from build123d import *

# Parameters (mm, degrees)
SKETCH1_W           = 101.6
SKETCH1_H           = 17.78
SKETCH1_R           = 3.96875
BOSS_EXTRUDE1_DEPTH = 33.02
SKETCH2_R           = 2.4892
CUT_EXTRUDE1_DEPTH  = 17.78
SKETCH3_R           = 4.064
CUT_EXTRUDE2_DEPTH  = 4.826
CUT_EXTRUDE3_DEPTH  = 109.300548475
FILLET1_R           = 2.54
SKETCH6_W           = 13.97
SKETCH6_H           = 22.86
SKETCH6_W_2         = 10.94852006
SKETCH6_H_2         = 22.718450652
CUT_EXTRUDE4_DEPTH  = 106.921350067
FILLET2_R           = 2.54
FILLET3_R           = 1.27


with BuildPart() as part:
    # Sketch1 → Boss-Extrude1 (new body)
    with BuildSketch(Plane(origin=(0, 0, 0), x_dir=(1, 0, 0), z_dir=(0, 1, 0))):
        with Locations((50.8, 8.89)):
            Rectangle(SKETCH1_W, SKETCH1_H)
        with Locations(Location((76.2, 8.89, 0), (0, 0, 270))):
            Circle(SKETCH1_R, mode=Mode.SUBTRACT)
        with Locations(Location((25.4, 8.89, 0), (0, 0, 270))):
            Circle(SKETCH1_R, mode=Mode.SUBTRACT)
    extrude(amount=-BOSS_EXTRUDE1_DEPTH)

    # Sketch2 → Cut-Extrude1 (cut)
    with BuildSketch(Plane.XY):
        with Locations((63.5, -16.51)):
            Circle(SKETCH2_R)
        with Locations((12.7, -16.51)):
            Circle(SKETCH2_R)
    extrude(amount=-CUT_EXTRUDE1_DEPTH, mode=Mode.SUBTRACT)

    # Sketch3 → Cut-Extrude2 (cut)
    with BuildSketch(Plane.XY):
        with Locations((63.5, -16.51)):
            Circle(SKETCH3_R)
        with Locations((12.7, -16.51)):
            Circle(SKETCH3_R)
    extrude(amount=-CUT_EXTRUDE2_DEPTH, mode=Mode.SUBTRACT)

    # Sketch5 → Cut-Extrude3 (cut, through all)
    with BuildSketch(Plane.XY):
        with BuildLine():
            Line((12.7, -5.150774674), (12.7, 0))
            Line((12.7, 0), (0, 0))
            Line((0, 0), (0, -33.02))
            Line((0, -33.02), (12.7, -33.02))
            Line((12.7, -33.02), (12.7, -27.869225326))
            ThreePointArc((12.7, -27.869225326), (12.37660211, -27.022558659), (11.571111111, -26.607089178))
            ThreePointArc((11.571111111, -26.607089178), (2.54, -16.51), (11.571111111, -6.412910822))
            ThreePointArc((11.571111111, -6.412910822), (12.37660211, -5.997441341), (12.7, -5.150774674))
        make_face()
        with BuildLine():
            Line((88.9, -5.150774674), (88.9, 0))
            Line((88.9, 0), (101.6, 0))
            Line((101.6, 0), (101.6, -33.02))
            Line((101.6, -33.02), (88.9, -33.02))
            Line((88.9, -33.02), (88.9, -27.869225326))
            ThreePointArc((88.9, -27.869225326), (89.22339789, -27.022558659), (90.028888889, -26.607089178))
            ThreePointArc((90.028888889, -26.607089178), (99.06, -16.51), (90.028888889, -6.412910822))
            ThreePointArc((90.028888889, -6.412910822), (89.22339789, -5.997441341), (88.9, -5.150774674))
        make_face()
    extrude(amount=-CUT_EXTRUDE3_DEPTH, mode=Mode.SUBTRACT)

    # Fillet1
    fillet1_edges = [part.edges().sort_by_distance(p)[0] for p in [
        (12.7, -33.02, -8.89),
        (12.7, 0, -8.89),
        (88.9, 0, -8.89),
        (88.9, -33.02, -8.89),
    ]]
    fillet(fillet1_edges, radius=FILLET1_R)

    # Sketch6 → Cut-Extrude4 (cut, through all)
    with BuildSketch(Plane.XY):
        with BuildLine():
            Line((19.05, -21.9075), (19.05, -11.1125))
            ThreePointArc((19.05, -11.1125), (19.793948776, -9.316448776), (21.59, -8.5725))
            Line((21.59, -8.5725), (31.75, -8.5725))
            Line((31.75, -8.5725), (31.75, -5.08))
            Line((31.75, -5.08), (54.61, -5.08))
            ThreePointArc((54.61, -5.08), (56.406051224, -5.823948776), (57.15, -7.62))
            Line((57.15, -7.62), (57.15, -25.4))
            ThreePointArc((57.15, -25.4), (56.406051224, -27.196051224), (54.61, -27.94))
            Line((54.61, -27.94), (31.75, -27.94))
            Line((31.75, -27.94), (31.75, -24.4475))
            Line((31.75, -24.4475), (21.59, -24.4475))
            ThreePointArc((21.59, -24.4475), (19.793948776, -23.703551224), (19.05, -21.9075))
        make_face()
        with Locations((76.835, -16.51)):
            Rectangle(SKETCH6_W, SKETCH6_H)
        with Locations((94.37426003, -16.51)):
            Rectangle(SKETCH6_W_2, SKETCH6_H_2)
    extrude(amount=-CUT_EXTRUDE4_DEPTH, mode=Mode.SUBTRACT)

    # Fillet2
    fillet2_edges = [part.edges().sort_by_distance(p)[0] for p in [
        (69.85, -5.08, -8.89),
        (83.82, -27.94, -8.89),
        (83.82, -5.08, -8.89),
        (69.85, -27.94, -8.89),
    ]]
    fillet(fillet2_edges, radius=FILLET2_R)

    # Fillet3
    fillet3_edges = [part.edges().sort_by_distance(p)[0] for p in [
        (31.75, -24.4475, -8.89),
        (31.75, -8.5725, -8.89),
        (31.75, -5.08, -8.89),
        (31.75, -27.94, -8.89),
    ]]
    fillet(fillet3_edges, radius=FILLET3_R)


solid = part.part
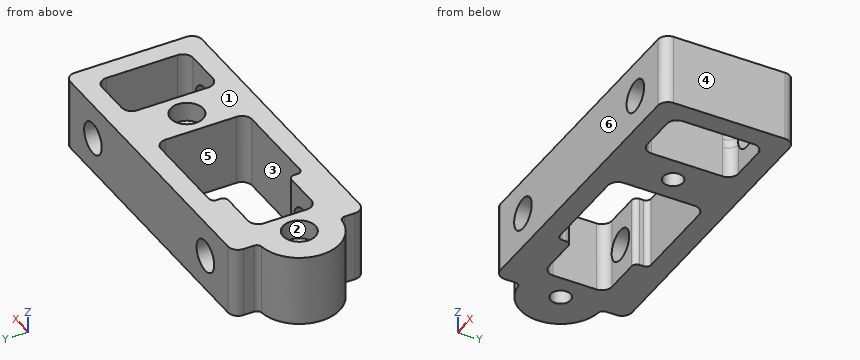
Geometry check sheet. Reference: the model listing, model coordinates, mm. Face numbers are marked on the shaded views. A direction names the side the tool comes from. Give positions to 0.01 mm unless a question says otherwise; leave off trailing zeros. Order: outer loops, then holes, each group sorted by start corner. A loop starts at its lowest first (then second) coordinate and runs counter-clockwise, first axis right, second up. Notation, with made-up numbers: M 88.5,63.5 L 100.5,63.5 A17 ccw 100.5,88.5 Z; hole C -10.5,8.5 d11. An arc over 180 degrees is marked long. Use a Markdown table: item, result.
Item 1: Section check C-C (x = 37.5). Record the cut outline in (y, z), and give its area (3 significant figures).
Answers follow:
| item | result |
|---|---|
| outline | M -33.02,-17.78 L -27.94,-17.78 L -27.94,0 L -33.02,0 Z; M -5.08,-17.78 L 0,-17.78 L 0,0 L -5.08,0 Z |
| area | 181 mm2 |
Item 2: Section check D-D (y = -23.5). Record the cut outline in (x, z), and give its area (3 significant figures).
Answers follow:
| item | result |
|---|---|
| outline | M 5.33,-17.78 L 19.61,-17.78 L 19.61,0 L 5.33,0 Z; M 57.15,-17.78 L 69.85,-17.78 L 69.85,0 L 57.15,0 Z; M 83.82,-17.78 L 88.9,-17.78 L 88.9,0 L 83.82,0 Z |
| area | 570 mm2 |
Item 3: Draft check along X on the marked faces 4, 5 and 6. Enter one of: +X half, -X half, draft (parallel to the pull), parting line (faces both ways), or undercut.
Answers follow:
| item | result |
|---|---|
| face 4 | +X half |
| face 5 | undercut |
| face 6 | draft |
Item 4: Section check A-A (x = 25.4). Record the cut outline in (y, z).
Answers follow:
| item | result |
|---|---|
| outline | M -33.02,-17.78 L -24.45,-17.78 L -24.45,-12.86 L -33.02,-12.86 Z; M -33.02,-4.92 L -24.45,-4.92 L -24.45,0 L -33.02,0 Z; M -8.57,-17.78 L 0,-17.78 L 0,-12.86 L -8.57,-12.86 Z; M -8.57,-4.92 L 0,-4.92 L 0,0 L -8.57,0 Z |
Item 5: Material ranges on line 1 along X through (y, z) = (-28, -8.89); line 2 along X through (y, z) = (-16.5, -6); line 3 along Y through (x, z) = (23.5, -4.5), recorded low to high.
Answers follow:
| item | result |
|---|---|
| line 1 | x = 12.7 to 21.43, 29.37 to 72.23, 80.17 to 88.9 |
| line 2 | x = 2.54 to 10.21, 15.19 to 19.05, 57.15 to 61.01, 65.99 to 69.85, 83.82 to 88.9 |
| line 3 | y = -33.02 to -24.45, -8.57 to 0 |
Item 6: Section check B-B (y = -16.51). Record the cut outline in (x, z).
Answers follow:
| item | result |
|---|---|
| outline | M 2.54,-17.78 L 10.21,-17.78 L 10.21,-4.83 L 8.64,-4.83 L 8.64,0 L 2.54,0 Z; M 15.19,-17.78 L 19.05,-17.78 L 19.05,0 L 16.76,0 L 16.76,-4.83 L 15.19,-4.83 Z; M 57.15,-17.78 L 61.01,-17.78 L 61.01,-4.83 L 59.44,-4.83 L 59.44,0 L 57.15,0 Z; M 65.99,-17.78 L 69.85,-17.78 L 69.85,0 L 67.56,0 L 67.56,-4.83 L 65.99,-4.83 Z; M 83.82,-17.78 L 88.9,-17.78 L 88.9,0 L 83.82,0 Z |
Item 7: Depth check by flat-ended pin: P1, Ø1.3, axis at y = -3.5, z = -11, coming from the -X side; P2, Ø8, axis at x = 12.7, y = -16.51, coming from the +Z side; P3, Ø4, axis at y = -23.5, z = -4, coming from the -X side. Enter the tip coordinate at first touch or a pass-through.
Answers follow:
| item | result |
|---|---|
| P1 | stops at x = 12.7 |
| P2 | stops at z = -4.83 |
| P3 | stops at x = 3.85 |
Item 8: Tool access check on the marked faces 1, 2 and 3. Record the directions out of +Z, -Z, +X, -X, +Y, -Y that give a thin tool (end or side, any length) a straight path to the whole face; none if there is none.
Answers follow:
| item | result |
|---|---|
| face 1 | +Z, +X, -X, +Y, -Y |
| face 2 | +Z |
| face 3 | +Z, -Z |
